Can you work these out from the model? Positions are in its coordinate system, mm. A direction names the side the tool comes from. Round coordinates to 2 decimals unless told otherwise and drop trailing zeros. Order: outer loops, then holes, each group sorted by start corner. A loop starts at its lowest first (then second) coordinate and runs counter-clockwise, first axis right, second up. Notation, with made-up numbers: M -22.5,3 L 2.5,3 A17 cw 2.5,26 Z; hole C 71.25,29.5 d4. An arc over 180 degrees is marked long. Answer as CSV lines item,"result". Start each with the question number.
from build123d import *

# Parameters (mm, degrees)
F1_DEPTH = 6


with BuildPart() as f1:
    # F0 (on Top) → F1 (new body)
    with BuildSketch(Plane.XY):
        with BuildLine():
            Line((-135, 21.9318206776), (-135, -38.0681793224))
            Line((-135, -38.0681793224), (-54, -38.0681793224))
            Line((-54, -38.0681793224), (-39, -38.0681793224))
            Line((-39, -38.0681793224), (-39, 6.9318206776))
            Line((-39, 6.9318206776), (-9, 6.9318206776))
            Line((-9, 6.9318206776), (-9, 18.9318206776))
            Line((-9, 18.9318206776), (-9, 33.9318206776))
            Line((-9, 33.9318206776), (-75, 33.9318206776))
            Line((-75, 33.9318206776), (-76, 33.9318206776))
            Line((-76, 33.9318206776), (-76, 46.9318206776))
            Line((-76, 46.9318206776), (-122.4432589807, 46.9318206776))
            ThreePointArc((-122.4432589807, 46.9318206776), (-131.6844515136, 35.9199562309), (-135, 21.9318206776))
        make_face()
        Polygon((-39, 6.9318206776), (-39, -38.0681793224), (-9, 6.9318206776), align=None)
        Polygon((9, 6.9318206776), (39, -38.0681793224), (39, 6.9318206776), align=None)
        with BuildLine():
            Line((54, -38.0681793224), (135, -38.0681793224))
            Line((135, -38.0681793224), (135, 21.9318206776))
            ThreePointArc((135, 21.9318206776), (131.6844515136, 35.9199562309), (122.4432589807, 46.9318206776))
            Line((122.4432589807, 46.9318206776), (76, 46.9318206776))
            Line((76, 46.9318206776), (76, 33.9318206776))
            Line((76, 33.9318206776), (75, 33.9318206776))
            Line((75, 33.9318206776), (9, 33.9318206776))
            Line((9, 33.9318206776), (9, 18.9318206776))
            Line((9, 18.9318206776), (9, 6.9318206776))
            Line((9, 6.9318206776), (39, 6.9318206776))
            Line((39, 6.9318206776), (39, -38.0681793224))
            Line((39, -38.0681793224), (54, -38.0681793224))
        make_face()
        with BuildLine():
            Line((-39, -38.0681793224), (-54, -38.0681793224))
            Line((-54, -38.0681793224), (-54, -44.0681793224))
            Line((-54, -44.0681793224), (-51.28125, -44.0681793224))
            ThreePointArc((-51.28125, -44.0681793224), (-44.5628777893, -42.2507556443), (-39, -38.0681793224))
        make_face()
        Polygon((-54, -38.0681793224), (-135, -38.0681793224), (-54, -44.0681793224), align=None)
        with BuildLine():
            Line((54, -44.0681793224), (54, -38.0681793224))
            Line((54, -38.0681793224), (39, -38.0681793224))
            ThreePointArc((39, -38.0681793224), (44.5628777893, -42.2507556443), (51.28125, -44.0681793224))
            Line((51.28125, -44.0681793224), (54, -44.0681793224))
        make_face()
        Polygon((54, -44.0681793224), (135, -38.0681793224), (54, -38.0681793224), align=None)
        Polygon((75, 33.9318206776), (75, 46.9318206776), (-75, 46.9318206776), (-75, 33.9318206776), (-9, 33.9318206776), (0, 33.9318206776), (9, 33.9318206776), align=None)
        Polygon((22.5, 62.9270896316), (22.5, 71.9318206776), (2.5, 71.9318206776), (2.5, 67.9318206776), (-2.5, 67.9318206776), (-2.5, 71.9318206776), (-22.5, 71.9318206776), (-22.5, 62.9270896316), align=None)
        with BuildLine():
            ThreePointArc((-110.5953234954, 52.3550821231), (-116.8058887661, 50.2695670793), (-122.4432589807, 46.9318206776))
            Line((-122.4432589807, 46.9318206776), (-76, 46.9318206776))
            Line((-76, 46.9318206776), (-76, 60.0429317887))
            Line((-76, 60.0429317887), (-110.5953234954, 52.3550821231))
        make_face()
        with BuildLine():
            Line((76, 46.9318206776), (122.4432589807, 46.9318206776))
            ThreePointArc((122.4432589807, 46.9318206776), (116.8058887661, 50.2695670793), (110.5953234954, 52.3550821231))
            Line((110.5953234954, 52.3550821231), (76, 60.0429317887))
            Line((76, 60.0429317887), (76, 46.9318206776))
        make_face()
        Polygon((-75, 46.9318206776), (75, 46.9318206776), (75, 60.2651540109), (22.5, 71.9318206776), (22.5, 62.9270896316), (-22.5, 62.9270896316), (-22.5, 71.9318206776), (-75, 60.2651540109), align=None)
        Polygon((-9, 18.9318206776), (9, 18.9318206776), (9, 33.9318206776), (0, 33.9318206776), (-9, 33.9318206776), align=None)
    extrude(amount=F1_DEPTH)


solid = f1.part
(1) If I drill on line 1 along X through (y, z) = (41.5, 2.75); line 2 along X through (y, z) = (37, 2.8); line 3 along X through (y, z) = (14, 2.1), over which ranges is the centre line in solid material (lowest first)?
(2) I want a section at A-A on y = -29.5. Write out the boundary of the cut face in (x, z).
(3) For faces 5 (the flat face through (-75, 47, 3)), 6 (the flat face through (93.93, -41.11, 2.96)), 7 (the flat face through (-9, 13, 3)), which set-ups out of +Z, -Z, +X, -X, +Y, -Y let a thin tool reach every point of the face, with its end or its side?
(4) If we mould it in two halves opening along X, with no side actions, what happens to faces 1 (the flat face through (49.117, 66.017, 2.958)), 2 (the flat face through (76, 47, 3)), 3 (the cylindrical face through (-127.96, 41.66, 2.96)), 4 (the flat face through (-76, 47, 3))? For each: +X half, -X half, draft (parallel to the pull), parting line (faces both ways), or undercut.
(5) I'm going to push flat-ended pins straight in: P1, Ø3, axis at y = 49.5, z = 3.5, coming from the +X side; P2, Ø0.8, axis at x = 75.5, z = 3.5, coming from the +Y side; P3, Ø3, axis at x = -1, z = 2, coming from the -Y side. Where does each tip first touch, or does it pass through?
(6) I want a section at B-B on y = 55. Write out the boundary of the cut face in (x, z), and give its area (3 significant figures).
(7) I want a section at C-C on y = -13.5. Write out the boundary of the cut face in (x, z).
(8) I want a section at D-D on x = -61.5. Write out the boundary of the cut face in (y, z).
From the geometry:
1,line 1,"-128.09 to -76, -75 to 75, 76 to 128.09"
1,line 2,"-131.12 to -76, -75 to 75, 76 to 131.12"
1,line 3,"-135 to -9, 9 to 135"
2,outline,"M -135,0 L -33.29,0 L -33.29,6 L -135,6 Z; M 33.29,0 L 135,0 L 135,6 L 33.29,6 Z"
3,face 5,"+Z, -Z, +Y"
3,face 6,"+Z, -Z, +X, -Y"
3,face 7,"+Z, -Z, -Y"
4,face 1,"+X half"
4,face 2,"undercut"
4,face 3,"-X half"
4,face 4,"undercut"
5,P1,"x = 120.91"
5,P2,"y = 33.93"
5,P3,"y = 18.93"
6,outline,"M -98.69,0 L -76,0 L -76,6 L -98.69,6 Z; M -75,0 L 75,0 L 75,6 L -75,6 Z; M 76,0 L 98.69,0 L 98.69,6 L 76,6 Z"
6,area,"1,170 mm²"
7,outline,"M -135,0 L -22.62,0 L -22.62,6 L -135,6 Z; M 22.62,0 L 135,0 L 135,6 L 22.62,6 Z"
8,outline,"M -43.51,0 L 63.27,0 L 63.27,6 L -43.51,6 Z"
